```python
from build123d import *

# Parameters (mm, degrees)
F1_DEPTH = 45
F2_W     = 114
F2_H     = 22
F3_DEPTH = 50
F5_DEPTH = 45
F6_R     = 3
F8_DEPTH = 5
F10_D    = 5.5


with BuildPart() as f1:
    # F0 (on Front) → F1 (new body)
    with BuildSketch(Plane.XZ):
        Polygon((0, 5), (0, 0), (160, 0), (160, 5), (140, 5), (140, 30), (20, 30), (20, 5), align=None)
    extrude(amount=F1_DEPTH)

    # F2 (on face) → F3 (cut)
    with BuildSketch(Plane.XZ.offset(45)):
        with Locations((80, 16)):
            Rectangle(F2_W, F2_H)
    extrude(amount=-F3_DEPTH, mode=Mode.SUBTRACT)

    # F4 (on face) → F5 (join, through all)
    with BuildSketch(Plane.XZ.offset(45)):
        with BuildLine():
            ThreePointArc((29.5, 5), (27.5961940777, 9.5961940777), (23, 11.5))
            Line((23, 11.5), (23, 5))
            Line((23, 5), (29.5, 5))
        make_face()
        with BuildLine():
            Line((23, 27), (23, 20.5))
            ThreePointArc((23, 20.5), (27.5961940777, 22.4038059223), (29.5, 27))
            Line((29.5, 27), (23, 27))
        make_face()
        with BuildLine():
            Line((137, 27), (130.5, 27))
            ThreePointArc((130.5, 27), (132.4038059223, 22.4038059223), (137, 20.5))
            Line((137, 20.5), (137, 27))
        make_face()
        with BuildLine():
            ThreePointArc((137, 11.5), (132.4038059223, 9.5961940777), (130.5, 5))
            Line((130.5, 5), (137, 5))
            Line((137, 5), (137, 11.5))
        make_face()
    extrude(amount=-F5_DEPTH)

    # F6
    f6_edges = [f1.edges().sort_by_distance(p)[0] for p in [
        (140, -22.5, 5),
        (20, -22.5, 5),
    ]]
    fillet(f6_edges, radius=F6_R)

    # F7 (on face) → F8 (cut, through all)
    with BuildSketch(Plane(origin=(0, 0, 0), x_dir=(1, 0, 0), z_dir=(0, 0, -1))):
        with BuildLine():
            ThreePointArc((12.6, 35), (10, 37.6), (7.4, 35))
            Line((7.4, 35), (7.4, 10))
            ThreePointArc((7.4, 10), (10, 7.4), (12.6, 10))
            Line((12.6, 10), (12.6, 35))
        make_face()
        with BuildLine():
            ThreePointArc((152.6, 35), (150, 37.6), (147.4, 35))
            Line((147.4, 35), (147.4, 10))
            ThreePointArc((147.4, 10), (150, 7.4), (152.6, 10))
            Line((152.6, 10), (152.6, 35))
        make_face()
    extrude(amount=-F8_DEPTH, mode=Mode.SUBTRACT)

    # F10 (through all)
    with Locations(Plane.XZ.offset(45)):
        with Locations((24.4142135624, 25.5857864376), (24.4142135624, 6.4142135624), (135.5857864376, 6.4142135624), (135.5857864376, 25.5857864376)):
            Hole(F10_D / 2)


solid = f1.part
```
Source: CAD feature listing. Evaluate the final solid. Frame: model axes, mm. A direction names the side the tool comes from. Round coordinates to 2 decimals unless told otherwise and drop trailing zeros. Loops run counter-clockwise (first coordinate to the right, second up) from the corner with the lowest first, then second, coordinate; pieces in that order, holes last. Notation, with made-up numbers: M 10,78 L 47,78 A16 ccw 47,101 Z; hole C 57.5,-34.75 d5. An arc over 180 degrees is marked long. Put each result on its own line as item: value.
(1) Section A-A, the plane x = 59. Return loops of the section in (y, z).
Solutions:
outline: M -45,0 L 0,0 L 0,5 L -45,5 Z; M -45,27 L 0,27 L 0,30 L -45,30 Z
(2) Ray query, line 1 (X direction, y = -6, z = 17.5); line 2 (X direction, y = -18.5, z = 6.5); line 3 (X direction, y = -10.5, z = 7.25). Return the intervals inside material, ascending. Write a range as [from, to].
Solutions:
line 1: [20, 23], [137, 140]
line 2: [19.6, 21.67], [27.16, 29.32], [130.68, 132.84], [138.33, 140.4]
line 3: [19.9, 21.79], [27.03, 29.1], [130.9, 132.97], [138.21, 140.1]
(3) Section B-B, the plane y = -13.5. State how many separate pieces and enclosed holes the cut face has, and give its area (3 significant figures).
Solutions:
separate pieces: 3
enclosed holes: 5
area: 1,280 mm²
(4) Section D-D, the plane y = -3.5. Return loops of the section in (x, z), and give its area (3 significant figures).
Solutions:
outline: M 0,0 L 160,0 L 160,5 L 143,5 A3 cw 140,8 L 140,30 L 20,30 L 20,8 A3 cw 17,5 L 0,5 Z; hole C 24.41,6.41 d5.5; hole C 24.41,25.59 d5.5; hole M 23,11.5 A6.5 cw 29.5,5 L 130.5,5 A6.5 cw 137,11.5 L 137,20.5 A6.5 cw 130.5,27 L 29.5,27 A6.5 cw 23,20.5 Z; hole C 135.59,6.41 d5.5; hole C 135.59,25.59 d5.5
area: 1,330 mm²
(5) Section C-C, the plane z = 16. Return loops of the section in (x, y).
Solutions:
outline: M 20,-45 L 23,-45 L 23,0 L 20,0 Z; M 137,-45 L 140,-45 L 140,0 L 137,0 Z
(6) Pull-direction query (Y, two-part tool) for faces 1 (the face through (7, -22, 5)), 2 (the face through (80, 0, 4)), 3 (the face through (12.6, -22, 2)); classes: released by +Y, released by -Y, zero draft, split by the parting line, or undercut.
Solutions:
face 1: zero draft
face 2: released by +Y
face 3: undercut
(7) First-contact query: pin 1 (1.5 mm diameter, centred on x = 67.5, y = -24.5, fed in from -Z); pin 2 (6.5 mm diameter, centred on y = -14, z = 20, fed in from +X); pin 3 (7 mm diameter, centred on y = -33.5, z = 14, fed in from -X); pin 4 (8.5 mm diameter, centred on x = 4.5, y = -27.5, fed in from +Z). Flat tips, straight axial feed; report the tip coordinate or a pass-through.
Solutions:
pin 1: z = 0
pin 2: x = 140
pin 3: x = 20
pin 4: z = 5
(8) Access query for faces 4 (the face through (79, -23, 27)), 5 (the face through (147.4, -23, 2)), 6 (the face through (140, -22, 19)). Directions: +Z, -Z, +X, -X, +Y, -Y. A direction counts if a zero-diameter tool reaches every point of the face in a straight line with its end or side. Return the directions, or none.
Solutions:
face 4: +Y, -Y
face 5: +Z, -Z
face 6: +Z, +X, +Y, -Y
